```python
from build123d import *

# Parameters (mm, degrees)
F1_DEPTH = 12.7


with BuildPart() as f1:
    # F0 (on Front) → F1 (new body)
    with BuildSketch(Plane.XZ):
        with BuildLine():
            Line((0, 8.153695), (0, 0))
            Line((0, 0), (12.7, 0))
            Line((12.7, 0), (12.7, 8.153695))
            Line((12.7, 8.153695), (9.525, 8.153695))
            ThreePointArc((9.525, 8.153695), (6.35, 4.978695), (3.175, 8.153695))
            Line((3.175, 8.153695), (0, 8.153695))
        make_face()
        with BuildLine():
            ThreePointArc((12.7, 8.153695), (6.35, 14.503695), (0, 8.153695))
            Line((0, 8.153695), (3.175, 8.153695))
            ThreePointArc((3.175, 8.153695), (6.35, 11.328695), (9.525, 8.153695))
            Line((9.525, 8.153695), (12.7, 8.153695))
        make_face()
    extrude(amount=F1_DEPTH)


solid = f1.part
```
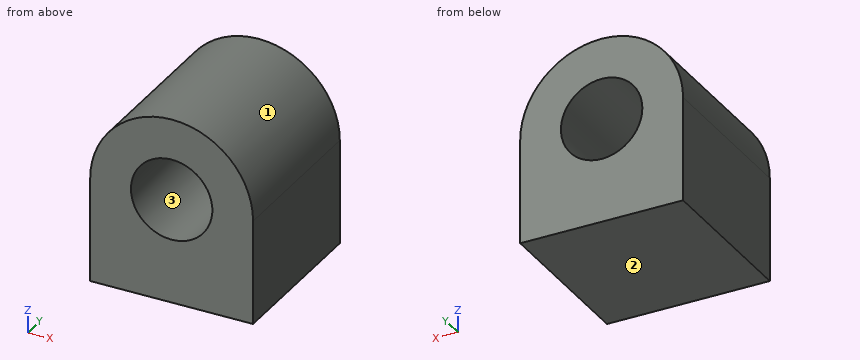
Read the model definition and answer for the solid it produces. Units are mm, in the model's axes. Face numbers are marked on the shaded views. Coordinates: 2 decimals unless noted, no trailing zeros. Loops run counter-clockwise (first coordinate to the right, second up) from the corner with the lowest first, then second, coordinate; pieces in that order, holes last.
(1) The mould has two halves that part along X. Classify the marked faces 1, 2 and 3: released by +X, released by -X, zero draft, split by the parting line, or undercut.
Solution:
face 1: split by the parting line
face 2: zero draft
face 3: undercut
(2) The part is cut by section D-D (x = 11.25). Determine the outline of the cut face in (y, z), and give its area (3 significant figures).
Solution:
outline: (-12.7, 0) - (0, 0) - (0, 12.19) - (-12.7, 12.19) - close
area: 155 mm2
(3) The part is cut by section B-B (z = 9). Determine the outline of the cut face in (x, y).
Solution:
outline: (0.06, -12.7) - (3.29, -12.7) - (3.29, 0) - (0.06, 0) - close; (9.41, -12.7) - (12.64, -12.7) - (12.64, 0) - (9.41, 0) - close
(4) Flat-ended cylindrical pins translate along their axes: pin 1 Ø4 at (y, z) = (-3, 12) entering from +X; pin 2 Ø2 at (x, y) = (2.5, -7.5) entering from +Z; pin 3 Ø5 at (x, y) = (3.5, -7.5) entering from +Z. Find the tip coordinate at first contact, or state that the pin passes through.
Solution:
pin 1: stops at x = 12.43
pin 2: stops at z = 13.83
pin 3: stops at z = 14.49
(5) The part is cut by section C-C (y = -11). Determine the outline of the cut face in (x, z) (3 decimals), and give its area (3 significant figures).
Solution:
outline: (0, 0) - (12.7, 0) - (12.7, 8.154) arc R6.35 ccw to (0, 8.154) - close; hole circle Ø6.35 at (6.35, 8.154)
area: 135 mm2
(6) Consider line 1 along Z through (x, y) = (6.35, -9); line 2 along X through (y, z) = (-6.5, 6); line 3 along Z through (x, y) = (4.75, -4.5). Determine where each line is inside the solid, lowest interval first.
Solution:
line 1: z = 0 to 4.98, 11.33 to 14.5
line 2: x = 0 to 4.02, 8.68 to 12.7
line 3: z = 0 to 5.41, 10.9 to 14.3
(7) The part is cut by section A-A (x = 6.35). Determine the outline of the cut face in (y, z), and give its area (3 significant figures).
Solution:
outline: (-12.7, 0) - (0, 0) - (0, 4.98) - (-12.7, 4.98) - close; (-12.7, 11.33) - (0, 11.33) - (0, 14.5) - (-12.7, 14.5) - close
area: 104 mm2
